from build123d import *

# Parameters (mm, degrees)
LINEAR_AUSTRAGEN_D_NN1_DEPTH = 6


with BuildPart() as part:
    # Skizze1 → Linear-Austragen-Dünn1 (new, symmetric)
    with BuildSketch(Plane.XY):
        with BuildLine():
            Line((-240, 11.8), (240, 11.8))
            ThreePointArc((240, 11.8), (245.149960176, 10.616869133), (249.267195462, 7.304730541))
            Line((249.267195462, 7.304730541), (282.767195462, -35.195269459))
            ThreePointArc((282.767195462, -35.195269459), (283.895246845, -48.083801843), (272.526696959, -54.259790865))
            Line((272.526696959, -54.259790865), (-240.973303041, -11.759790865))
            ThreePointArc((-240.973303041, -11.759790865), (-251.789943431, 0.487066624), (-240, 11.8))
        make_face()
        with BuildLine():
            Line((-240, 11), (240, 11))
            ThreePointArc((240, 11), (244.800810333, 9.897081395), (248.638911024, 6.809494572))
            Line((248.638911024, 6.809494572), (282.138911024, -35.690505428))
            ThreePointArc((282.138911024, -35.690505428), (283.190484347, -47.705239006), (272.592683605, -53.462516908))
            Line((272.592683605, -53.462516908), (-240.907316395, -10.962516908))
            ThreePointArc((-240.907316395, -10.962516908), (-250.990625232, 0.454045158), (-240, 11))
        make_face(mode=Mode.SUBTRACT)
    extrude(amount=LINEAR_AUSTRAGEN_D_NN1_DEPTH, both=True)


solid = part.part
Work out the finished part from the listing and answer in its coordinate system (mm). A direction names the side the tool comes from. Round coordinates to 2 decimals unless told otherwise and drop trailing zeros. Order: outer loops, then holes, each group sorted by start corner. A loop starts at its lowest first (then second) coordinate and runs counter-clockwise, first axis right, second up. Notation, with made-up numbers: M 75,27 L 83,27 A32 cw 83,66 Z; hole C 79.5,86 d8. An arc over 180 degrees is marked long. Put each result on its own line as item: value. Start each with the question number.
Q1. A tool of negligible diameter and unlimited length cuts with its end or side. For faces 1 (the flat face through (265.15, -14.14, 0.08)), 2 (the cylindrical face through (245.08, 10.65, 0.08)), from which of +Z, -Z, +X, -X, +Y, -Y can it reach the whole face along a straight path? Write none if from no direction.
Q2. Straight lines are drawn through the part: L1, parallel to Y at x = -18, z = 5.25; L2, parallel to Y at x = 87.5, z = 3.25; L3, parallel to X at y = 3.5, z = 0.25. For each, find the intervals that lie inside material, in ascending order. Write a range as [from, to].
Q3. Section A-A, the plane z = 4 is taken. Write down the section's boundary in (x, y), and give its area (3 significant figures).
Q4. Section B-B, the plane x = -2.5 is taken. Write down the section's boundary in (y, z), and give its area (3 significant figures).
Q5. For a pull along X with two mould halves and no side action, classify faces 3 (the flat face through (19.44, -32.51, 0.08)), 4 (the cylindrical face through (-251.8, 0.2, 0.1)), 5 (the flat face through (-3, 11.8, 0)) as pulls with the +X half, pulls with the -X half, needs draft (parallel to the pull), parting line crosses it, or undercut.
Q6. Flat-ended cylindrical pins translate along their axes: pin 1 (6 mm diameter, centred on x = -118.5, z = -4.5, fed in from -Y); pin 2 (3.5 mm diameter, centred on x = -59, z = 1, fed in from -Y); pin 3 (5 mm diameter, centred on x = -134.5, z = -1, fed in from -Y). Find the tip coordinate at first contact, or state that the pin passes through.
Q7. Section C-C, the plane y = -5 is taken. Write down the section's boundary in (x, z).
Findings below:
1. face 1: +Z, -Z
1. face 2: +Z, -Z, +X, +Y
2. L1: y = [-30.21, -29.41], [11, 11.8]
2. L2: y = [-38.95, -38.14], [11, 11.8]
2. L3: x = [-251.27, -250.43], [251.25, 252.27]
3. outline: M -240.97,-11.76 L 272.53,-54.26 A11.8 ccw 282.77,-35.2 L 249.27,7.3 A11.8 ccw 240,11.8 L -240,11.8 A11.8 ccw Z; hole M -240.91,-10.96 L 272.59,-53.46 A11 ccw 282.14,-35.69 L 248.64,6.81 A11 ccw 240,11 L -240,11 A11 ccw Z
3. area: 897 mm^2
4. outline: M -31.5,-6 L -30.69,-6 L -30.69,6 L -31.5,6 Z; M 11,-6 L 11.8,-6 L 11.8,6 L 11,6 Z
4. area: 19.2 mm^2
5. face 3: undercut
5. face 4: pulls with the -X half
5. face 5: needs draft
6. pin 1: stops at y = -22.14
6. pin 2: stops at y = -26.97
6. pin 3: stops at y = -20.78
7. outline: M -250.69,-6 L -249.8,-6 L -249.8,6 L -250.69,6 Z; M 257.95,-6 L 258.97,-6 L 258.97,6 L 257.95,6 Z
